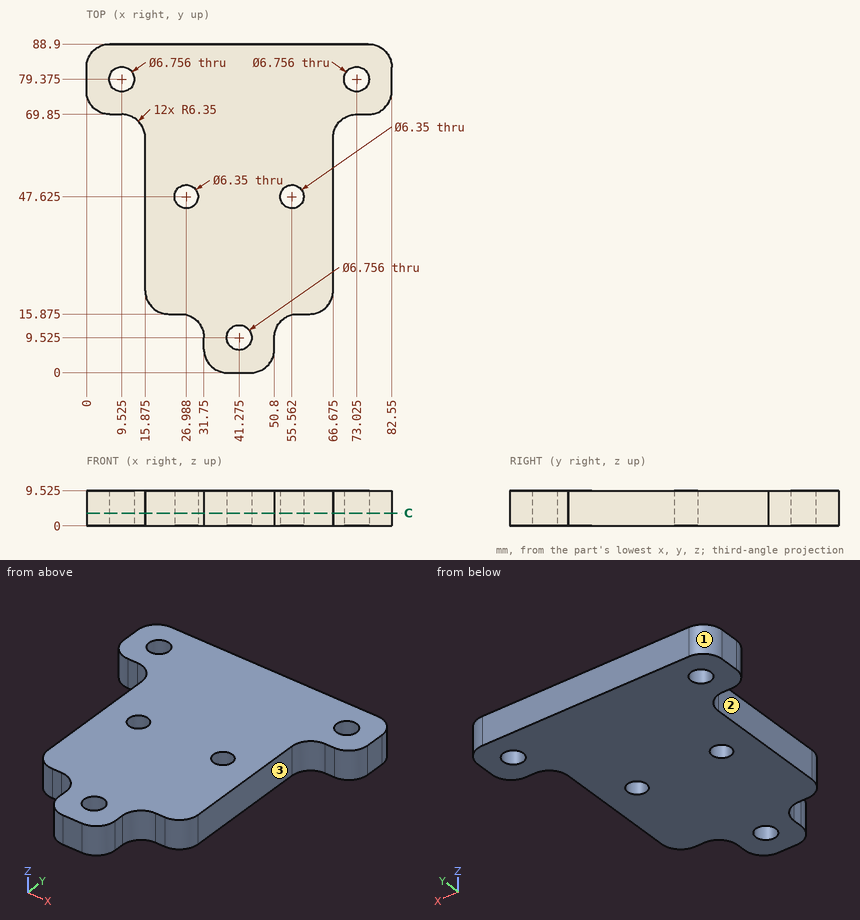
The drawing under review shows one solid part. Ordinate dimensions are in mm from its lowest x, y, z. A direction names the side the tool comes from. Round coordinates to 2 decimals unless told otherwise and drop trailing zeros. Use one line per item in the form item = value.
Q1. For line 1 (X direction, y = 78, z = 4.5); line 2 (X direction, y = 78.5, z = 4.5); line 3 (Y direction, x = 9.5, z = 6.75), list the stretches that pass through material, from the lowest coordinate up. Write a range as [from, to].
Answer key:
line_1 = [0, 6.44], [12.61, 69.94], [76.11, 82.55]
line_2 = [0, 6.26], [12.79, 69.76], [76.29, 82.55]
line_3 = [69.85, 76], [82.75, 88.9]
Q2. Tool access review of the marked faces 1, 2 and 3: name each direction out of +Z, -Z, +X, -X, +Y, -Y from which nothing blocks a thin tool from reaching the whole face with its end or side.
Answer key:
face_1 = +Z, -Z, -X, +Y
face_2 = +Z, -Z, -X, -Y
face_3 = +Z, -Z, +X, -Y
Q3. Insertion check: pin 1 Ø3.5 at (x, z) = (59, 7) entering from -Y (1 decimal); pin 2 Ø1 at (x, z) = (47.5, 3.5) entering from -Y (1 decimal); pin 3 Ø3 at (y, z) = (40.5, 3) entering from -X (1 decimal). Each pin has a flat end and moves straight along its axis. Give the tip position at first contact, or say it passes through.
Answer key:
pin_1 = 15.9
pin_2 = 0.5
pin_3 = 15.9
Q4. Consider section C-C (z = 3.5). State how many separate pieces and enclosed holes the cut face has, and give its area (3 significant figures).
Answer key:
separate_pieces = 1
enclosed_holes = 5
area = 4,410 mm2
